Could you check a few things on this model? Use its own coordinates, in mm. Face numbers are marked on the shaded views. A direction names the side the tool comes from. Give positions to 0.01 mm unless a question says otherwise; leave off trailing zeros. Loops run counter-clockwise (first coordinate to the right, second up) from the corner with the lowest first, then second, coordinate; pieces in that order, holes last. Notation, with made-up numbers: M 47.5,79.25 L 70.5,79.25 A16 cw 70.5,100.25 Z; hole C -7,11 d1. An arc over 180 degrees is marked long. Use a Markdown table: item, result. Add a question column.
1) Suppose I cut it at C-C on z = -39. List the corners of the cut face in (x, y) for me (3 decimals).
2) If I drill on line 1 along Z through (x, y) = (558.8, -0.6) (3 decimals); line 2 along Z through (x, y) = (311.15, -0.65) (3 decimals); line 3 along Y through (x, z) = (99.5, 274.5), over which ranges is the centre line in solid material (lowest first)? Write a range as [from, to].
3) Suppose I cut it at A-A on x = 429. List the corners of the cut face in (y, z) for me (3 decimals).
4) Which directions (+Z, -Z, +X, -X, +Y, -Y) give clear straight access to the entire face, cutting with the end or side of a thin tool? Please do the marked faces 1, 2 and 3.
5) Will these pins go through, and if not, where does the flat tip stop? pin 1 Ø6 at (x, z) = (234.95, 257.175) entering from -Y; pin 2 Ø4.5 at (x, z) = (234.95, 79.375) entering from -Y; pin 3 Ø10 at (x, y) = (210, -155.5) entering from -Z; pin 4 Ø8.5 at (x, y) = (311.15, -26.035) entering from +Z.
6) Suppose I cut it at B-B on y = -141. List the corners of the cut face in (x, z) for me (3 decimals), and give its area (3 significant figures).
```python
from build123d import *

# Parameters (mm, degrees)
F1_DEPTH  = 2.54
F2_R      = 2.579688
F2_R_2    = 3.175
F3_DEPTH  = 2.541
F4_W      = 552.45
F4_H      = 2.54
F5_DEPTH  = 257.175
F6_W      = 552.45
F6_H      = 2.54
F7_DEPTH  = 38.1
F8_R      = 2.579688
F9_DEPTH  = 259.716
F10_R     = 2.579688
F11_DEPTH = 561.976


with BuildPart() as f1:
    # F0 (on Front) → F1 (new body)
    with BuildSketch(Plane.XZ):
        Polygon((587.375, 336.55), (587.375, 447.675), (34.925, 447.675), (34.925, 336.55), (0, 336.55), (0, 0), (34.925, 0), (34.925, -114.3), (587.375, -114.3), (587.375, 0), (622.3, 0), (622.3, 336.55), align=None)
    extrude(amount=F1_DEPTH)

    # F2 (on face) → F3 (cut, through all)
    with BuildSketch(Plane(origin=(0, 0, 0), x_dir=(-1, 0, 0), z_dir=(0, 1, 0))):
        with Locations((-558.8, 434.975)):
            Circle(F2_R)
        with Locations((-558.8, 358.775)):
            Circle(F2_R)
        with Locations((-63.5, 358.775)):
            Circle(F2_R)
        with Locations((-63.5, 434.975)):
            Circle(F2_R)
        with Locations((-609.6, 316.70625)):
            Circle(F2_R_2)
        with Locations((-609.6, 168.275)):
            Circle(F2_R_2)
        with Locations((-609.6, 19.84375)):
            Circle(F2_R_2)
        with Locations((-12.7, 19.84375)):
            Circle(F2_R_2)
        with Locations((-12.7, 168.275)):
            Circle(F2_R_2)
        with Locations((-12.7, 316.70625)):
            Circle(F2_R_2)
        with Locations((-558.8, -22.225)):
            Circle(F2_R)
        with Locations((-558.8, -98.425)):
            Circle(F2_R)
        with Locations((-63.5, -98.425)):
            Circle(F2_R)
        with Locations((-63.5, -22.225)):
            Circle(F2_R)
        with Locations((-85.725, 257.175)):
            Circle(F2_R)
        with Locations((-536.575, 257.175)):
            Circle(F2_R)
        with Locations((-234.95, 257.175)):
            Circle(F2_R)
        with Locations((-387.35, 257.175)):
            Circle(F2_R)
        with Locations((-311.15, 257.175)):
            Circle(F2_R)
        with Locations((-158.75, 257.175)):
            Circle(F2_R)
        with Locations((-460.375, 257.175)):
            Circle(F2_R)
        with Locations((-460.375, 79.375)):
            Circle(F2_R)
        with Locations((-234.95, 79.375)):
            Circle(F2_R)
        with Locations((-158.75, 79.375)):
            Circle(F2_R)
        with Locations((-85.725, 79.375)):
            Circle(F2_R)
        with Locations((-387.35, 79.375)):
            Circle(F2_R)
        with Locations((-311.15, 79.375)):
            Circle(F2_R)
        with Locations((-536.575, 79.375)):
            Circle(F2_R)
    extrude(amount=-F3_DEPTH, mode=Mode.SUBTRACT)

    # F4 (on face) → F5 (join)
    with BuildSketch(Plane.XZ.offset(2.54)):
        with Locations((311.15, -113.03)):
            Rectangle(F4_W, F4_H)
    extrude(amount=F5_DEPTH)

    # F6 (on face) → F7 (join)
    with BuildSketch(Plane(origin=(0, 0, -114.3), x_dir=(1, 0, 0), z_dir=(0, 0, -1))):
        with Locations((311.15, 258.445)):
            Rectangle(F6_W, F6_H)
    extrude(amount=F7_DEPTH)

    # F8 (on face) → F9 (cut, through all)
    with BuildSketch(Plane.XZ.offset(259.715)):
        with Locations((311.15, -139.7)):
            Circle(F8_R)
        with Locations((558.8, -139.7)):
            Circle(F8_R)
        with Locations((63.5, -139.7)):
            Circle(F8_R)
    extrude(amount=-F9_DEPTH, mode=Mode.SUBTRACT)

    # F10 (on face) → F11 (cut, through all)
    with BuildSketch(Plane(origin=(0, 0, -114.3), x_dir=(1, 0, 0), z_dir=(0, 0, -1))):
        with Locations((311.15, 26.035)):
            Circle(F10_R)
        with Locations((558.8, 26.035)):
            Circle(F10_R)
        with Locations((63.5, 26.035)):
            Circle(F10_R)
    extrude(amount=-F11_DEPTH, mode=Mode.SUBTRACT)


solid = f1.part
```
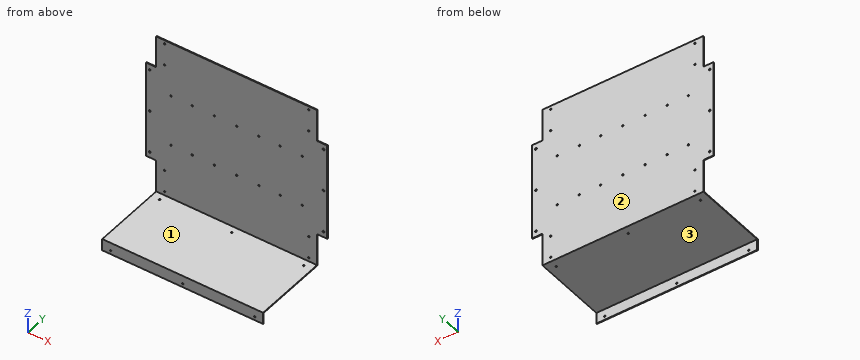
Answer block:
| question | item | result |
|---|---|---|
| 1 | outline | M 34.925,-2.54 L 587.375,-2.54 L 587.375,0 L 34.925,0 Z |
| 2 | line 1 | z = [-114.3, -101.005], [-95.845, -24.805], [-19.645, 356.195], [361.355, 432.395], [437.555, 447.675] |
| 2 | line 2 | z = [-114.3, 76.795], [81.955, 254.595], [259.755, 447.675] |
| 2 | line 3 | y = [-2.54, 0] |
| 3 | outline | M -259.715,-152.4 L -257.175,-152.4 L -257.175,-114.3 L 0,-114.3 L 0,447.675 L -2.54,447.675 L -2.54,-111.76 L -259.715,-111.76 Z |
| 4 | face 1 | +Z, +X, -X, -Y |
| 4 | face 2 | +Z, -Z, +X, -X, +Y |
| 4 | face 3 | -Z, +X, -X, +Y |
| 5 | pin 1 | stops at y = -2.54 |
| 5 | pin 2 | passes through |
| 5 | pin 3 | stops at z = -114.3 |
| 5 | pin 4 | stops at z = -111.76 |
| 6 | outline | M 34.925,-114.3 L 587.375,-114.3 L 587.375,-111.76 L 34.925,-111.76 Z |
| 6 | area | 1,400 mm^2 |
